from build123d import *

# Parameters (mm, degrees)
F1_DEPTH = 6
F2_R     = 19
F3_DEPTH = 30
F4_R     = 20
F5_DEPTH = 24
F6_R     = 16
F7_DEPTH = 60.001
F8_SIZE  = 1
F9_SIZE2 = 5
F9_SIZE  = 0.5


with BuildPart() as f1:
    # F0 (on Front) → F1 (new body)
    with BuildSketch(Plane.XZ):
        Polygon((24.248698, 0.025049), (12.102656, 21.012513), (-12.146042, 20.987464), (-24.248698, -0.025049), (-12.102656, -21.012513), (12.146042, -20.987464), align=None)
    extrude(amount=F1_DEPTH)

    # F2 (on face) → F3 (join)
    with BuildSketch(Plane.XZ.offset(6)):
        Circle(F2_R)
    extrude(amount=F3_DEPTH)

    # F4 (on face) → F5 (join)
    with BuildSketch(Plane(origin=(0, 0, 0), x_dir=(-1, 0, 0), z_dir=(0, 1, 0))):
        Circle(F4_R)
    extrude(amount=F5_DEPTH)

    # F6 (on face) → F7 (cut, through all)
    with BuildSketch(Plane(origin=(0, 24, 0), x_dir=(-1, 0, 0), z_dir=(0, 1, 0))):
        Circle(F6_R)
    extrude(amount=-F7_DEPTH, mode=Mode.SUBTRACT)

    # F8
    f8_edges = [f1.edges().sort_by_distance(p)[0] for p in [
        (20, 24, 0),
    ]]
    chamfer(f8_edges, length=F8_SIZE)

    # F9
    f9_edges = [f1.edges().sort_by_distance(p)[0] for p in [
        (-19, -36, 0),
    ]]
    chamfer(f9_edges, length=F9_SIZE, length2=F9_SIZE2)


solid = f1.part
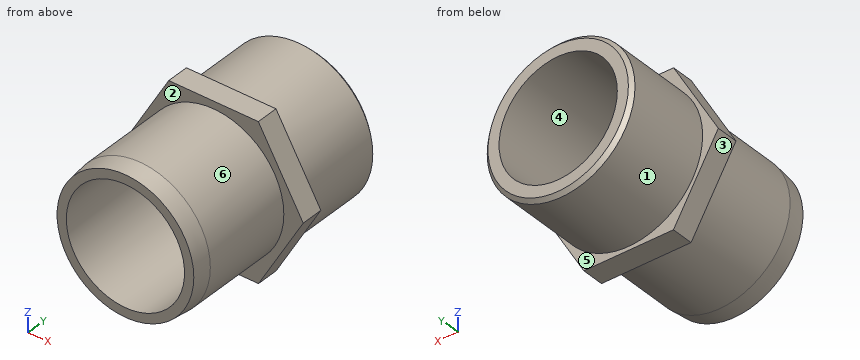
Input: part model. Units: mm. Frame: model coordinates. Face numbers are marked on the shaded views. A direction names the side the tool comes from. Round coordinates to 2 decimals unless told otherwise and drop trailing zeros. Write each loop counter-clockwise with the first axis right and the second up, starting at its lowest first coordinate (ties: lowest second). Pieces come first, ordered by that corner, then holes.
1) Reachability of the marked faces 1, 2 and 3 from +Z, -Z, +X, -X, +Y, -Y: full face, straight path, thin tool, end or side. Return the list, or none.
2) Ray query, L1, parallel to Z at x = 0, y = -19; L2, parallel to Z at x = -8.5, y = 17; L3, parallel to X at y = 12, z = 12.5. Return the intervals inside material, ascending.
3) Cut plane A-A (x = 0). Return the cut outline in (y, z).
4) Draft query along X for the marked faces 4, 5 and 6. Return one class per face: pulls with the +X half, pulls with the -X half, needs draft (parallel to the pull), parting line crosses it, or undercut.
5) Cut plane B-B (y = -7.5). Return the cut outline in (x, z).
6) Contact query for flat-ended pins moving along their axis: P1, Ø1.5, axis at y = -15.5, z = 10.5, coming from the -X side; P2, Ø3, axis at x = -16, y = -15.5, coming from the -Z side; P3, Ø2, axis at x = -11, y = 6, coming from the -Z side; P4, Ø5, axis at x = 5.5, z = 12, coming from the -Y side. Output: stop coordinate, or through.
Geometry says:
1. face 1: +Y
1. face 2: -Y
1. face 3: -Z, -X, +Y, -Y
2. L1: z = -19 to -16, 16 to 19
2. L2: z = -18.1 to -13.56, 13.56 to 18.1
2. L3: x = -15.61 to -9.99, 9.99 to 15.61
3. outline: (-36, -18.5) - (-31, -19) - (-6, -19) - (-6, -21) - (0, -21) - (0, -20) - (23, -20) - (24, -19) - (24, -16) - (-36, -16) - close; (-36, 16) - (24, 16) - (24, 19) - (23, 20) - (0, 20) - (0, 21) - (-6, 21) - (-6, 19) - (-31, 19) - (-36, 18.5) - close
4. face 4: undercut
4. face 5: needs draft
4. face 6: parting line crosses it
5. outline: circle Ø38 at (0, 0); hole circle Ø32 at (0, 0)
6. P1: stops at x = -16.31
6. P2: stops at z = -12.28
6. P3: stops at z = -17.32
6. P4: passes through
